from build123d import *

# Parameters (mm, degrees)
ESBO_O1_W                = 43
ESBO_O1_H                = 30
ESBO_O1_R                = 4.5
ESBO_O1_R_2              = 1.205837633
RESSALTO_EXTRUS_O1_DEPTH = 2
ESBO_O2_R                = 1.5
RESSALTO_EXTRUS_O2_DEPTH = 2


with BuildPart() as part:
    # Esboço1 → Ressalto-extrusão1 (new body)
    with BuildSketch(Plane(origin=(0, 0, 0), x_dir=(1, 0, 0), z_dir=(0, 1, 0))):
        Rectangle(ESBO_O1_W, ESBO_O1_H)
        Circle(ESBO_O1_R, mode=Mode.SUBTRACT)
        with Locations((7, 7)):
            Circle(ESBO_O1_R_2, mode=Mode.SUBTRACT)
        with Locations((-6, 6)):
            Circle(ESBO_O1_R_2, mode=Mode.SUBTRACT)
        with Locations((-8, 9)):
            Circle(ESBO_O1_R_2, mode=Mode.SUBTRACT)
        with Locations((-7, -7)):
            Circle(ESBO_O1_R_2, mode=Mode.SUBTRACT)
        with Locations((6, -6)):
            Circle(ESBO_O1_R_2, mode=Mode.SUBTRACT)
        with Locations((8, -9)):
            Circle(ESBO_O1_R_2, mode=Mode.SUBTRACT)
    extrude(amount=RESSALTO_EXTRUS_O1_DEPTH)

    # Esboço2 → Ressalto-extrusão2 (add)
    with BuildSketch(Plane.ZY.offset(21.5)):
        Polygon((15, 2), (15, 12), (-15, 8.089445099), (-15, 2), align=None)
        with Locations((-9, 6)):
            Circle(ESBO_O2_R, mode=Mode.SUBTRACT)
        with BuildLine():
            ThreePointArc((8.240400933, 8.233448591), (9.539925295, 8.339457279), (10.431505763, 7.388097368))
            ThreePointArc((10.431505763, 7.388097368), (11.835840488, 7.245540316), (12.5, 6))
            ThreePointArc((12.5, 6), (11.226651005, 4.51722243), (9.568494237, 5.551902632))
            ThreePointArc((9.568494237, 5.551902632), (8.567535869, 5.503694052), (7.759599067, 6.096551409))
            ThreePointArc((7.759599067, 6.096551409), (6.624037685, 5.937880054), (5.708151293, 6.62768319))
            ThreePointArc((5.708151293, 6.62768319), (3.55555397, 8.354444888), (6.291848707, 8.71231681))
            ThreePointArc((6.291848707, 8.71231681), (7.357982, 8.84665675), (8.240400933, 8.233448591))
        make_face(mode=Mode.SUBTRACT)
    ressalto_extrus_o2 = extrude(amount=-RESSALTO_EXTRUS_O2_DEPTH)

    # Espelhar1: Ressalto-extrusão2 across plane
    add(ressalto_extrus_o2.mirror(Plane(origin=(0, 0, 0), x_dir=(0, 0, 1), z_dir=(1, 0, 0))))


solid = part.part
Design review of the part built by this model. Coordinates are the model's own, in mm. A direction names the side the tool comes from. Coordinates: 2 decimals unless noted, no trailing zeros. Write each loop counter-clockwise with the first axis right and the second up, starting at its lowest first coordinate (ties: lowest second). Pieces come first, ordered by that corner, then holes. Notation, with made-up numbers: (-14.75, -7.75) - (-10.75, -7.75) arc R35 ccw to (-10.75, 25.25) - close; hole circle Ø3 at (89, -20.75). An arc over 180 degrees is marked (long way). Use one line per item in the form item = value.
Q1. Consider section B-B (y = 1.25). Write out the cut boundary in (x, z), plus the area to 3 significant figures.
Taken from the geometry:
outline = (-21.5, -15) - (21.5, -15) - (21.5, 15) - (-21.5, 15) - close; hole circle Ø2.41 at (-8, -9); hole circle Ø2.41 at (-7, 7); hole circle Ø2.41 at (-6, -6); hole circle Ø9 at (0, 0); hole circle Ø2.41 at (6, 6); hole circle Ø2.41 at (7, -7); hole circle Ø2.41 at (8, 9)
area = 1,200 mm^2
Q2. Insertion check: pin 1 Ø3 at (x, z) = (-7, 7) entering from +Y. The pin has a flat end and moves straight along its axis. Give the tip position at first contact, or say it passes through.
Taken from the geometry:
pin_1 = 2
Q3. Machinability: for faces 5 (the cylindrical face through (-20.51, 8.85, 7.34)), 6 (the flat face through (-20.514, 10.072, 0.21)), which of the approach directions +Z, -Z, +X, -X, +Y, -Y give a long, thin tool a straight path to every point of the face, cutting with its end or side? Answer none if there is none.
Taken from the geometry:
face_5 = +X, -X
face_6 = -Z, +X, -X, +Y
Q4. Consider section D-D (y = 10). Write out the cut boundary in (x, z).
Taken from the geometry:
outline = (-21.5, -0.34) - (-19.5, -0.34) - (-19.5, 15) - (-21.5, 15) - close; (19.5, -0.34) - (21.5, -0.34) - (21.5, 15) - (19.5, 15) - close
Q5. Consider section C-C (z = 1.5). Write out the cut boundary in (x, y), plus the area to 3 significant figures.
Taken from the geometry:
outline = (-21.5, 0) - (-4.24, 0) - (-4.24, 2) - (-19.5, 2) - (-19.5, 10.24) - (-21.5, 10.24) - close; (4.24, 0) - (21.5, 0) - (21.5, 10.24) - (19.5, 10.24) - (19.5, 2) - (4.24, 2) - close
area = 102 mm^2
Q6. Consider section A-A (x = 0). Write out the cut boundary in (y, z), plus the area to 3 significant figures.
Taken from the geometry:
outline = (0, -15) - (2, -15) - (2, -4.5) - (0, -4.5) - close; (0, 4.5) - (2, 4.5) - (2, 15) - (0, 15) - close
area = 42.0 mm^2
Q7. For probe 1 along X at (y, z) = (2.5, 0.25); probe 2 along Z at (x, y) = (-6, 0.85); probe 3 along X at (y, z) = (1.05, 0), list the stretches that pass through material, from the lowest coordinate up.
Taken from the geometry:
probe_1 = -21.5 to -19.5, 19.5 to 21.5
probe_2 = -15 to -7.21, -4.79 to 6.33, 7.67 to 15
probe_3 = -21.5 to -4.5, 4.5 to 21.5
Q8. The part is to be moulded in two halves that separate along Z. For faces 1 (the cylindrical face through (-20.514, 8.346, 9.522)), 2 (the flat face through (5, 1, 15)), 3 (the cylindrical face through (7.843, 0.986, 7.804)), 4 (the flat face through (-19.5, 6, 0)), say which applies: +Z half, -Z half, draft (parallel to the pull), parting line (faces both ways), or undercut.
Taken from the geometry:
face_1 = undercut
face_2 = +Z half
face_3 = undercut
face_4 = draft
